```python
from build123d import *

# Parameters (mm, degrees)
BOSS_EXTRUDE1_DEPTH = 60
FILLET1_R           = 1
SKETCH2_R           = 1.5
CUT_EXTRUDE1_DEPTH  = 40


with BuildPart() as part:
    # Sketch1 → Boss-Extrude1 (new body)
    with BuildSketch(Plane(origin=(0, 0, 0), x_dir=(0, 0, -1), z_dir=(1, 0, 0))):
        Polygon((0, 2), (0, 0), (12, 0), (12, 23), (25, 23), (25, 25), (22, 25), (10, 25), (10, 2), align=None)
    extrude(amount=BOSS_EXTRUDE1_DEPTH)

    # Fillet1
    fillet1_edges = [part.edges().sort_by_distance(p)[0] for p in [
        (30, 23, -12),
        (30, 0, -12),
        (30, 2, -10),
        (30, 25, -10),
    ]]
    fillet(fillet1_edges, radius=FILLET1_R)

    # Sketch2 → Cut-Extrude1 (cut)
    with BuildSketch(Plane(origin=(0, 25, 0), x_dir=(1, 0, 0), z_dir=(0, 1, 0))):
        with Locations(Location((10, 20, 0), (0, 0, 270))):
            Circle(SKETCH2_R)
        with Locations(Location((50, 20, 0), (0, 0, 270))):
            Circle(SKETCH2_R)
    extrude(amount=-CUT_EXTRUDE1_DEPTH, mode=Mode.SUBTRACT)


solid = part.part
```
The model under review builds one solid part; all positions refer to its coordinate system, in mm. A direction names the side the tool comes from. Round coordinates to 2 decimals unless told otherwise and drop trailing zeros. Order: outer loops, then holes, each group sorted by start corner. A loop starts at its lowest first (then second) coordinate and runs counter-clockwise, first axis right, second up. Notation, with made-up numbers: M 59.5,23.25 L 63.5,23.25 A21 cw 63.5,46.25 Z; hole C -24.5,53 d1. An arc over 180 degrees is marked long. Use a Markdown table: item, result.
1) Draft analysis for pull direction X (two halves, no side actions). For faces 1 (the face through (10.07, 24.01, -21.5)), 2 (the face through (0, 13.5, -11.5)), 3 (the face through (30, 1, 0)), state which applies: released by +X, released by -X, zero draft, split by the parting line, or undercut.
Report:
| item | result |
|---|---|
| face 1 | undercut |
| face 2 | released by -X |
| face 3 | zero draft |
2) Consider section A-A (x = 50). Write out the cut boundary in (y, z), then the cut area to 3 significant figures.
Report:
| item | result |
|---|---|
| outline | M 0,-11 A1 ccw 1,-12 L 22,-12 A1 cw 23,-13 L 23,-18.5 L 25,-18.5 L 25,-11 A1 ccw 24,-10 L 3,-10 A1 cw 2,-9 L 2,0 L 0,0 Z; M 23,-25 L 25,-25 L 25,-21.5 L 23,-21.5 Z |
| area | 90.0 mm^2 |
3) Insertion check: pin 1 (10 mm diameter, centred on x = 23, z = -4.5, fed in from +Y); pin 2 (9.5 mm diameter, centred on x = 31, z = -17.5, fed in from -Y); pin 3 (1.5 mm diameter, centred on x = 20.5, y = 11, fed in from -Z); pin 4 (1.8 mm diameter, centred on x = 50, z = -20, fed in from -Y). Each pin has a flat end and moves straight along its axis. Give the tip position at first contact, or say it passes through.
Report:
| item | result |
|---|---|
| pin 1 | y = 2.13 |
| pin 2 | y = 22.97 |
| pin 3 | z = -12 |
| pin 4 | through |
4) Consider section B-B (z = -20). Write out the cut boundary in (x, y).
Report:
| item | result |
|---|---|
| outline | M 0,23 L 8.5,23 L 8.5,25 L 0,25 Z; M 11.5,23 L 48.5,23 L 48.5,25 L 11.5,25 Z; M 51.5,23 L 60,23 L 60,25 L 51.5,25 Z |
5) Wall thickness on line 1 along X through (y, z) = (23.5, -20); line 2 along Y through (x, z) = (18, -21.25); line 3 along Y through (x, z) = (46, -3.5): over which ranges is each line inside the solid? List them lowest first. Write a range as [from, to].
Report:
| item | result |
|---|---|
| line 1 | [0, 8.5], [11.5, 48.5], [51.5, 60] |
| line 2 | [23, 25] |
| line 3 | [0, 2] |
6) Consider section D-D (z = -7.75). Write out the cut boundary in (x, y).
Report:
| item | result |
|---|---|
| outline | M 0,0 L 60,0 L 60,2 L 0,2 Z |
7) Tool access review of faces 4 (the face through (30, 24, -25)), 5 (the face through (30, 2, -5)), 6 (the face through (30, 11, -12)): name each direction out of +Z, -Z, +X, -X, +Y, -Y from which nothing blocks a thin tool from reaching the whole face with its end or side.
Report:
| item | result |
|---|---|
| face 4 | -Z, +X, -X, +Y, -Y |
| face 5 | +Z, +X, -X, +Y |
| face 6 | -Z, +X, -X, -Y |
8) Consider section C-C (x = 31). Write out the cut boundary in (y, z).
Report:
| item | result |
|---|---|
| outline | M 0,-11 A1 ccw 1,-12 L 22,-12 A1 cw 23,-13 L 23,-25 L 25,-25 L 25,-11 A1 ccw 24,-10 L 3,-10 A1 cw 2,-9 L 2,0 L 0,0 Z |
